Model file for the job. Use its own axes, mm. A direction names the side the tool comes from. Round coordinates to 2 decimals unless told otherwise and drop trailing zeros. Write each loop counter-clockwise with the first axis right and the second up, starting at its lowest first coordinate (ties: lowest second). Pieces come first, ordered by that corner, then holes.
```python
from build123d import *

# Parameters (mm, degrees)
F0_W         = 95.3032001853
F0_H         = 78.1703665853
F1_DEPTH     = 25.4
F2_T         = -2.54
F3_W         = 5.7767406106
F3_H         = 42.3835292459
F4_DEPTH     = 3.175
F5_W         = 5.7767406106
F5_H         = 42.3835292459
F6_DEPTH     = 3.175
F7_T1_DEPTH  = 66.0677355788
F7_T3_DEPTH  = 66.8133734297
F7_T8_DEPTH  = 84.3633291385
F7_T13_DEPTH = 84.3633291385
F8_T1_DEPTH  = 33.1027333037
F8_T6_ANGLE  = 211.2479562886
F8_T12_ANGLE = 207.4140629141
F8_T15_DEPTH = 67.9213053823


# Not quite as in the source:
# - a fillet or chamfer that OpenCascade refuses, or shapes differently, is made with other operations: its cross-section is extruded or revolved along the edge and cut away or added


with BuildPart() as f1:
    # F0 (on Front) → F1 (new body)
    with BuildSketch(Plane.XZ):
        with Locations((47.6516000926, 39.0851832926)):
            Rectangle(F0_W, F0_H)
    extrude(amount=F1_DEPTH)

    # F2
    f2_openings = [f1.faces().sort_by_distance(p)[0] for p in [
        (95.3032, -12.7, 39.085183),
    ]]
    offset(amount=F2_T, openings=f2_openings)

    # F3 (on face) → F4 (join)
    with BuildSketch(Plane(origin=(0, 0, 0), x_dir=(-1, 0, 0), z_dir=(0, 1, 0))):
        with Locations((-77.4001292884, 39.3448248506)):
            Rectangle(F3_W, F3_H)
    extrude(amount=F4_DEPTH)

    # F5 (on face) → F6 (join)
    with BuildSketch(Plane(origin=(0, 3.175, 0), x_dir=(-1, 0, 0), z_dir=(0, 1, 0))):
        Polygon((-74.5117589831, 60.5365894735), (-74.5117589831, 18.1530602276), (-19.4716006517, 18.1530602276), (-19.4716006517, 60.6743656099), (-80.2884995937, 60.6743656099), (-80.2884995937, 60.5365894735), align=None)
        with Locations((-77.4001292884, 39.3448248506)):
            Rectangle(F5_W, F5_H)
    extrude(amount=F6_DEPTH)

    # F7: fillet of radius 5.08 on 3 edges, made by hand

    # F7_s2 → F7_t1 (cut)
    with BuildSketch(Plane.XY.offset(6.3798451294)):
        with BuildLine():
            ThreePointArc((19.4716006517, 6.35), (21.3410803596, 4.0428865162), (24.180886691, 3.175))
            Line((24.180886691, 3.175), (19.4716006517, 3.175))
            Line((19.4716006517, 3.175), (19.4716006517, 6.35))
        make_face()
    extrude(amount=F7_T1_DEPTH, mode=Mode.SUBTRACT)

    # F7_s4 → F7_t3 (cut)
    with BuildSketch(Plane.YZ.offset(7.6983855535)):
        with BuildLine():
            ThreePointArc((3.175, 22.8623462669), (4.0428865162, 20.0225399355), (6.35, 18.1530602276))
            Line((6.35, 18.1530602276), (3.175, 18.1530602276))
            Line((3.175, 18.1530602276), (3.175, 22.8623462669))
        make_face()
    extrude(amount=F7_T3_DEPTH, mode=Mode.SUBTRACT)


with BuildPart() as f7_tool6:
    # F7_s7 → F7_t8 (new body)
    with BuildSketch(Plane.YZ.offset(7.6983855535)):
        with BuildLine():
            ThreePointArc((6.35, 60.6743656099), (4.0428865162, 58.804885902), (3.175, 55.9650795706))
            Line((3.175, 55.9650795706), (3.175, 60.6743656099))
            Line((3.175, 60.6743656099), (6.35, 60.6743656099))
        make_face()
    extrude(amount=F7_T8_DEPTH)

    split(bisect_by=Plane.XY.offset(60.5365894735), keep=Keep.TOP)


with BuildPart() as f1_1:
    add(f1.part)

    # F7_t5: cut F7_tool6
    add(f7_tool6.part, mode=Mode.SUBTRACT)


with BuildPart() as f7_tool11:
    # F7_s12 → F7_t13 (new body)
    with BuildSketch(Plane.YZ.offset(7.6983855535)):
        with BuildLine():
            ThreePointArc((6.35, 60.6743656099), (4.0428865162, 58.804885902), (3.175, 55.9650795706))
            Line((3.175, 55.9650795706), (3.175, 60.6743656099))
            Line((3.175, 60.6743656099), (6.35, 60.6743656099))
        make_face()
    extrude(amount=F7_T13_DEPTH)

    split(bisect_by=Plane.YZ.offset(74.5117589831), keep=Keep.BOTTOM)


with BuildPart() as f1_2:
    add(f1_1.part)

    # F7_t10: cut F7_tool11
    add(f7_tool11.part, mode=Mode.SUBTRACT)

    # F8: fillet of radius 5.08 on 2 edges, made by hand

    # F8_s2 → F8_t1 (join)
    with BuildSketch(Plane.XY.offset(22.8623462669)):
        with BuildLine():
            ThreePointArc((69.4317589831, 3.175), (73.0238614316, 1.6871024484), (74.5117589831, -1.905))
            Line((74.5117589831, -1.905), (74.5117589831, 3.175))
            Line((74.5117589831, 3.175), (69.4317589831, 3.175))
        make_face()
    extrude(amount=F8_T1_DEPTH)


with BuildPart() as f8_tool4:
    # F8_s5 → F8_t6 (revolve)
    with BuildSketch(Plane.XY.offset(22.8623462668)):
        with BuildLine():
            ThreePointArc((69.4317589831, 3.175), (73.0238614316, 1.6871024484), (74.5117589831, -1.905))
            Line((74.5117589831, -1.905), (74.5117589831, 3.175))
            Line((74.5117589831, 3.175), (69.4317589831, 3.175))
        make_face()
    revolve(axis=Axis((74.5117589831, 8.2549999999, 22.8623462668), (1, 0, 0)), revolution_arc=F8_T6_ANGLE)

    split(bisect_by=Plane.XZ.offset(-6.35), keep=Keep.TOP)

    split(bisect_by=Plane.XY.offset(18.1530602276), keep=Keep.TOP)


with BuildPart() as f1_3:
    add(f1_2.part)

    # F8_t3: union F8_tool4
    add(f8_tool4.part)


with BuildPart() as f8_tool10:
    # F8_s11 → F8_t12 (revolve)
    with BuildSketch(Plane.XY.offset(55.9650795707)):
        with BuildLine():
            ThreePointArc((69.4317589831, 3.175), (73.0238614316, 1.6871024484), (74.5117589831, -1.905))
            Line((74.5117589831, -1.905), (74.5117589831, 3.175))
            Line((74.5117589831, 3.175), (69.4317589831, 3.175))
        make_face()
    revolve(axis=Axis((74.5117589831, 8.2549999999, 55.9650795707), (-1, 0, 0)), revolution_arc=F8_T12_ANGLE)

    split(bisect_by=Plane.XZ.offset(-6.35), keep=Keep.TOP)

    split(bisect_by=Plane.XY.offset(60.5365894735), keep=Keep.BOTTOM)


with BuildPart() as f1_4:
    add(f1_3.part)

    # F8_t9: union F8_tool10
    add(f8_tool10.part)

    # F8_s16 → F8_t15 (cut)
    with BuildSketch(Plane.XY.offset(5.4530602276)):
        with BuildLine():
            ThreePointArc((75.2084995937, 6.35), (78.8006020422, 4.8621024484), (80.2884995937, 1.27))
            Line((80.2884995937, 1.27), (80.2884995937, 6.35))
            Line((80.2884995937, 6.35), (75.2084995937, 6.35))
        make_face()
    extrude(amount=F8_T15_DEPTH, mode=Mode.SUBTRACT)


solid = f1_4.part
```
1) Wall check: probe 1 along Y at (x, z) = (20, 67); probe 2 along Z at (x, y) = (26, -14); probe 3 along X at (y, z) = (-21.5, 42). Give the ranges that are in metal, low to high.
2) Cut at A-A on x = 54.5. List the corners of the cut face in (y, z) (3 decimals), and give its area (3 significant figures).
3) Cut at D-D on x = 13. List the corners of the cut face in (y, z).
4) Cut at B-B on y = -6. List the corners of the cut face in (x, z), and give its area (3 significant figures).
5) Which spindle directions (+Z, -Z, +X, -X, +Y, -Y) get a long thin tool onto all of the face, cutting with end or side? Do faces 4 (the face through (47.812, 4.067, 58.84)), 5 (the face through (44.1, 4.02, 20.06)), 6 (the face through (48, -2.54, 40)), 7 (the face through (21.306, 4.067, 39.116)). Say none if no direction does.
6) Flat gauge pins, fed straight in: pin 1 Ø10 at (y, z) = (-16.5, 27) entering from +X; pin 2 Ø1.9 at (x, y) = (72.5, 2.5) entering from -Z. Where does each tip first touch, or does it go through?
7) Pull direction Y, two halves, no side cores. Call faces 1 (the face through (47, -25.4, 40)), 2 (the face through (95.303, -2, 39)), 3 (the face through (2.54, -13, 39)): released by +Y, released by -Y, zero draft, split by the parting line, or undercut.
Result sheet:
1. probe 1: y = -25.4 to -22.86, -2.54 to 0
1. probe 2: z = 0 to 2.54, 75.63 to 78.17
1. probe 3: x = 0 to 2.54
2. outline: (-25.4, 0) - (0, 0) - (0, 78.17) - (-25.4, 78.17) - close; (3.175, 22.862) arc R5.08 ccw to (6.35, 18.153) - (6.35, 60.674) arc R5.08 ccw to (3.175, 55.965) - close; hole (-22.86, 2.54) - (-2.54, 2.54) - (-2.54, 75.63) - (-22.86, 75.63) - close
2. area: 627 mm2
3. outline: (-25.4, 0) - (0, 0) - (0, 78.17) - (-25.4, 78.17) - close; hole (-22.86, 2.54) - (-2.54, 2.54) - (-2.54, 75.63) - (-22.86, 75.63) - close
4. outline: (0, 0) - (95.3, 0) - (95.3, 2.54) - (2.54, 2.54) - (2.54, 75.63) - (95.3, 75.63) - (95.3, 78.17) - (0, 78.17) - close
4. area: 670 mm2
5. face 4: +Z, -X
5. face 5: -Z, -X
5. face 6: +X
5. face 7: +Z, -Z, -X
6. pin 1: stops at x = 2.54
6. pin 2: stops at z = 18.43
7. face 1: released by -Y
7. face 2: zero draft
7. face 3: undercut
